Check sheet for the modelled part. Datum: model origin and axes. Units: mm. A direction names the side the tool comes from. Give positions to 0.01 mm unless a question says otherwise; leave off trailing zeros. Order: outer loops, then holes, each group sorted by start corner. A loop starts at its lowest first (then second) coordinate and runs counter-clockwise, first axis right, second up. Notation, with made-up numbers: (45.25, 76.5) - (104.25, 76.5) arc R11 cw to (104.25, 96.5) - close; hole circle Ø11 at (66.5, 17.25). An arc over 180 degrees is marked (long way). Answer in a Markdown table with one row per item.
from build123d import *

# Parameters (mm, degrees)
F1_DEPTH = 25.4
F2_T     = -2.54


with BuildPart() as f1:
    # F0 (on Front) → F1 (new body)
    with BuildSketch(Plane.XZ):
        Polygon((21.808967, -17.473448), (0, 37.180346), (-40.166995, -14.075698), (-42.829655, -17.473448), align=None)
        Polygon((-42.829655, -17.473448), (-40.166995, -14.075698), (-47.980445, -4.553055), (-51.23793, -7.225862), align=None)
    extrude(amount=F1_DEPTH)

    # F2
    f2_openings = [f1.faces().sort_by_distance(p)[0] for p in [
        (-8.148417, -25.4, 0.40127),
        (-8.148417, 0, 0.40127),
    ]]
    offset(amount=F2_T, openings=f2_openings)


solid = f1.part
(1) Gauge pin test, flat ends, axial feed: P1, Ø1.5, axis at y = -14.5, z = 12, coming from the +X side; P2, Ø10, axis at y = -14, z = 20.5, coming from the -X side; P3, Ø1, axis at y = -16, z = 20, coming from the +X side. Record the tip position at first contact, or that the pin passes through.
Geometry says:
| item | result |
|---|---|
| P1 | x = 10.35 |
| P2 | x = -16.99 |
| P3 | x = 7.06 |
(2) Cross-section at D-D, the plane z = 9.5. Record the cut outline in (x, y).
Geometry says:
| item | result |
|---|---|
| outline | (-21.69, -25.4) - (-18.46, -25.4) - (-18.46, 0) - (-21.69, 0) - close; (8.31, -25.4) - (11.05, -25.4) - (11.05, 0) - (8.31, 0) - close |
(3) Cross-section at A-A, the plane y = -22. Record the cut outline in (x, z).
Geometry says:
| item | result |
|---|---|
| outline | (-51.24, -7.23) - (-42.83, -17.47) - (21.81, -17.47) - (0, 37.18) - (-40.17, -14.08) - (-47.98, -4.55) - close; hole (-37.61, -14.93) - (18.06, -14.93) - (-0.72, 32.14) - close |
(4) Cross-section at B-B, the plane z = -11.5. Record the cut outline in (x, y).
Geometry says:
| item | result |
|---|---|
| outline | (-47.73, -25.4) - (-42.28, -25.4) - (-42.28, 0) - (-47.73, 0) - close; (-38.15, -25.4) - (-34.92, -25.4) - (-34.92, 0) - (-38.15, 0) - close; (16.69, -25.4) - (19.43, -25.4) - (19.43, 0) - (16.69, 0) - close |
(5) Access from +Z, -Z, +X, -X, +Y, -Y to the whole of each face (thin tool, end or side, straight path). Record for faces 4 (the flat face through (-10, -13, -14.933)), 5 (the flat face through (-47.09, -12.52, -12.28)), 6 (the flat face through (-44.02, -12.52, -9.38)).
Geometry says:
| item | result |
|---|---|
| face 4 | +Y, -Y |
| face 5 | -Z, -X, +Y, -Y |
| face 6 | +Z, +Y, -Y |
(6) Mould release check, pull along X, two halves, no side actions. Record for faces 1 (the flat face through (-49.586, -12.522, -5.871)), 2 (the flat face through (-19.802, -12.522, 11.911)), 3 (the flat face through (11.057, -12.522, 9.471)): pulls with the +X half, pulls with the -X half, needs draft (parallel to the pull), parting line crosses it, or undercut.
Geometry says:
| item | result |
|---|---|
| face 1 | pulls with the -X half |
| face 2 | undercut |
| face 3 | pulls with the +X half |
(7) Cross-section at C-C, the plane x = 16. Record the cut outline in (y, z), then the cut area to 3 significant figures.
Geometry says:
| item | result |
|---|---|
| outline | (-25.4, -17.47) - (0, -17.47) - (0, -14.93) - (-25.4, -14.93) - close; (-25.4, -9.77) - (0, -9.77) - (0, -2.92) - (-25.4, -2.92) - close |
| area | 239 mm² |
(8) Thickness scan on L1, parallel to X at y = -14.25, z = -7; L2, parallel to X at y = -24, z = -12.5; L3, parallel to X at y = -5, z = 28. Record the ranges inside material, lowest first.
Geometry says:
| item | result |
|---|---|
| L1 | -50.96 to -45.97, -34.62 to -31.4, 14.89 to 17.63 |
| L2 | -46.91 to -41.46, -38.93 to -35.71, 17.09 to 19.82 |
| L3 | -7.19 to -3.97, 0.93 to 3.66 |
